Model file for the job. Use its own axes, mm. Face numbers are marked on the shaded views. A direction names the side the tool comes from. Give positions to 0.01 mm unless a question says otherwise; leave off trailing zeros. Loops run counter-clockwise (first coordinate to the right, second up) from the corner with the lowest first, then second, coordinate; pieces in that order, holes last. Notation, with made-up numbers: M 6.25,-12 L 13.25,-12 A16 cw 13.25,-6 Z; hole C -27,87 d10. An arc over 180 degrees is marked long. Answer in a Markdown table with one row per item.
Autodesk Inventor part; units mm, degrees
ref_plane "YZ Plane" through (0, 0, 0) normal (1, 0, 0) x (0, 1, 0)
ref_plane "XZ Plane" through (0, 0, 0) normal (0, 1, 0) x (-1, 0, 0)
ref_plane "XY Plane" through (0, 0, 0) normal (0, 0, 1) x (1, 0, 0)
sketch "Skizze1" plane through (0, 0, 0) normal (0, 0, 1) x (1, 0, 0)
  circle A0 centre (0, 0) radius 13.75
  circle A1 centre (0, 0) radius 5
  line L0 (0, 13.75) -> (0, -13.75) construction
  circle A2 centre (0, 9) radius 4
  circle A3 centre (0, 9) radius 2.25
  circle A4 centre (0, -9) radius 4
  circle A5 centre (0, -9) radius 2.25
  line L1 (-13.75, 0) -> (13.75, 0) construction
  circle A6 centre (0, 0) radius 2.75
  circle A7 centre (0, 0) radius 3.5
  dimension "d0" = 27.5
  dimension "d1" = 10
  dimension "d4" = 8
  dimension "d5" = 18
  dimension "d6" = 4.5
  dimension "d7" = 5.5
  dimension "d14" = 7
extrude "Extrusion1" add sketch "Skizze1" against normal blind 5 contours A0 | A1 | A4 | A2 | A6 | A7
extrude "Extrusion2" cut sketch "Skizze1" against normal blind 3 contours A4 | A2
extrude "Extrusion3" add sketch "Skizze1" along normal blind 24 contours A1
extrude "Extrusion4" add sketch "Skizze1" along normal blind 24 contours A7
properties part number "Schalter_Basis_rund"
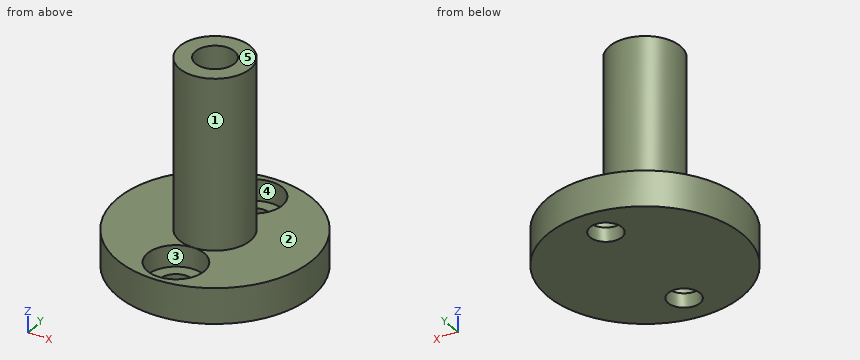
Q1. Saw through at D-D (x = 10.5). Give the cut face in (y, z).
Reported:
| item | result |
|---|---|
| outline | M -8.88,-5 L 8.88,-5 L 8.88,0 L -8.88,0 Z |
Q2. Probe probe 1 along Y at (x, z) = (0, -1); probe 2 along Y at (x, z) = (0, -3.7); probe 3 along Y at (x, z) = (0, 20.75). List the from-to ranges inside material, lowest first.
Reported:
| item | result |
|---|---|
| probe 1 | -13.75 to -13, -5 to 5, 13 to 13.75 |
| probe 2 | -13.75 to -11.25, -6.75 to 6.75, 11.25 to 13.75 |
| probe 3 | -5 to -2.75, 2.75 to 5 |
Q3. 3-axis set-ups, long thin cutter, end or side, ignore diameter. For the marked faces 4 and 5: which of +Z, -Z, +X, -X, +Y, -Y reach the whole face in a straight line?
Reported:
| item | result |
|---|---|
| face 4 | +Z |
| face 5 | +Z, +X, -X, +Y, -Y |
Q4. Saw through at C-C (y = -10). Give the cut face in (x, z).
Reported:
| item | result |
|---|---|
| outline | M -9.44,-5 L -2.02,-5 L -2.02,-3 L -3.87,-3 L -3.87,0 L -9.44,0 Z; M 2.02,-5 L 9.44,-5 L 9.44,0 L 3.87,0 L 3.87,-3 L 2.02,-3 Z |
Q5. Saw through at B-B (z = 22). Give the cut face in (x, y).
Reported:
| item | result |
|---|---|
| outline | C 0,0 d10; hole C 0,0 d5.5 |
Q6. Mould opens along X. For the marked faces 1, 2 and 3 say: released by +X, released by -X, zero draft, split by the parting line, or undercut.
Reported:
| item | result |
|---|---|
| face 1 | split by the parting line |
| face 2 | zero draft |
| face 3 | undercut |
Q7. Drop flat-ended pins along their axis: pin 1 (7 mm diameter, centred on x = 0, y = 9, fed in from -Z); pin 2 (6.5 mm diameter, centred on x = 0, y = -9, fed in from +Z); pin 3 (10 mm diameter, centred on y = -7, z = 19.5, fed in from +X); pin 4 (3 mm diameter, centred on x = 9, z = -1.5, fed in from +Y). Give the stop position or say it passes through.
Reported:
| item | result |
|---|---|
| pin 1 | z = -5 |
| pin 2 | z = -3 |
| pin 3 | x = 4.58 |
| pin 4 | y = 11.52 |
Q8. Saw through at A-A (y = 0). Give the cut face in (x, z), and give its area (4 significant figures).
Reported:
| item | result |
|---|---|
| outline | M -13.75,-5 L 13.75,-5 L 13.75,0 L 5,0 L 5,24 L 2.75,24 L 2.75,0 L -2.75,0 L -2.75,24 L -5,24 L -5,0 L -13.75,0 Z |
| area | 245.5 mm² |
